```python
from build123d import *

# Parameters (mm, degrees)
SKETCH1_R           = 10
BOSS_EXTRUDE1_DEPTH = 10
SKETCH2_R           = 9.5
CUT_EXTRUDE1_DEPTH  = 6
SKETCH3_R           = 5
CUT_EXTRUDE2_DEPTH  = 11
CUT_EXTRUDE4_DEPTH  = 11
FILLET1_R           = 2
M4_TAPPED_HOLE1_D   = 3


with BuildPart() as part:
    # Sketch1 → Boss-Extrude1 (new body)
    with BuildSketch(Plane(origin=(0, 0, 0), x_dir=(1, 0, 0), z_dir=(0, 1, 0))):
        with BuildLine():
            Line((-14.758244484, -9.68540076), (-11.496273776, -137.792727273))
            ThreePointArc((-11.496273776, -137.792727273), (0, -149), (11.496273776, -137.792727273))
            Line((11.496273776, -137.792727273), (14.758244484, -9.68540076))
            ThreePointArc((14.758244484, -9.68540076), (15.434637081, -8.136753315), (17, -7.5))
            Line((17, -7.5), (17, 7.5))
            ThreePointArc((17, 7.5), (13.764151011, 8.182075624), (11.078928313, 10.112237509))
            ThreePointArc((11.078928313, 10.112237509), (0, 15), (-11.078928313, 10.112237509))
            ThreePointArc((-11.078928313, 10.112237509), (-13.764151011, 8.182075624), (-17, 7.5))
            Line((-17, 7.5), (-17, -7.5))
            ThreePointArc((-17, -7.5), (-15.434637081, -8.136753315), (-14.758244484, -9.68540076))
        make_face()
        Circle(SKETCH1_R, mode=Mode.SUBTRACT)
    extrude(amount=BOSS_EXTRUDE1_DEPTH)

    # Sketch2 → Cut-Extrude1 (cut)
    with BuildSketch(Plane(origin=(0, 0, 0), x_dir=(1, 0, 0), z_dir=(0, 1, 0))):
        with Locations((0, -137.5)):
            Circle(SKETCH2_R)
    extrude(amount=CUT_EXTRUDE1_DEPTH, mode=Mode.SUBTRACT)

    # Sketch3 → Cut-Extrude2 (cut, through all)
    with BuildSketch(Plane(origin=(0, 0, 0), x_dir=(-1, 0, 0), z_dir=(0, -1, 0))):
        with Locations((0, -137.5)):
            Circle(SKETCH3_R)
    extrude(amount=-CUT_EXTRUDE2_DEPTH, mode=Mode.SUBTRACT)

    # Sketch4 → Cut-Extrude4 (cut, through all)
    with BuildSketch(Plane(origin=(0, 0, 0), x_dir=(1, 0, 0), z_dir=(0, 1, 0))):
        with BuildLine():
            Line((-7.90050824, -82.580601653), (-6.96789079, -119.207272727))
            ThreePointArc((-6.96789079, -119.207272727), (0, -126), (6.96789079, -119.207272727))
            Line((6.96789079, -119.207272727), (7.90050824, -82.580601653))
            ThreePointArc((7.90050824, -82.580601653), (0, -74.476363636), (-7.90050824, -82.580601653))
        make_face()
        with BuildLine():
            Line((-9.376393506, -24.618181818), (-8.443776056, -61.244852893))
            ThreePointArc((-8.443776056, -61.244852893), (0, -69.476363636), (8.443776056, -61.244852893))
            Line((8.443776056, -61.244852893), (9.376393506, -24.618181818))
            ThreePointArc((9.376393506, -24.618181818), (0, -15), (-9.376393506, -24.618181818))
        make_face()
    extrude(amount=CUT_EXTRUDE4_DEPTH, mode=Mode.SUBTRACT)

    # Fillet1
    fillet1_edges = [part.edges().sort_by_distance(p)[0] for p in [
        (17, 5, -7.5),
        (17, 5, 7.5),
        (-17, 5, 7.5),
        (-17, 5, -7.5),
    ]]
    fillet(fillet1_edges, radius=FILLET1_R)

    # M4 Tapped Hole1 (through all)
    with Locations(Plane.ZY.offset(17)):
        with Locations((0, 5)):
            Hole(M4_TAPPED_HOLE1_D / 2)


solid = part.part
```
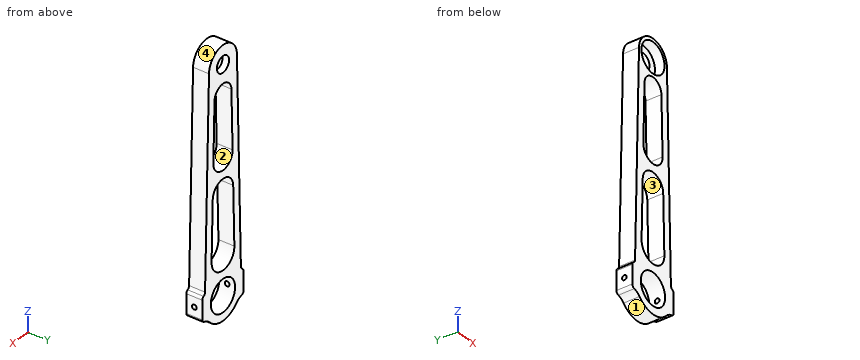
Geometry check sheet. Reference: the model listing, model coordinates, mm. Face numbers are marked on the shaded views. A direction names the side the tool comes from. Coordinates: 2 decimals unless noted, no trailing zeros. Order: outer loops, then holes, each group sorted by start corner. A loop starts at its lowest first (then second) coordinate and runs counter-clockwise, first axis right, second up.
Item 1: Scan lines: line 1 along Y through (x, z) = (-12, 0); line 2 along Z through (x, y) = (4, 9.5); line 3 along Z through (x, y) = (4.5, 6.5). Record each from-to range of solid material in increasing order.
Item 2: Tool access check on the marked faces 1 and 2. Record the directions out of +Z, -Z, +X, -X, +Y, -Y that give a thin tool (end or side, any length) a straight path to the whole face; none if there is none.
Item 3: Section check A-A (x = 0). Enter the section's corners in (y, z).
Item 4: Section check B-B (z = 0). Enter the section's corners in (x, y), plus the area to 3 significant figures.
Item 5: Section check D-D (x = 13). Enter the section's corners in (y, z).
Item 6: Mould release check, pull along X, two halves, no side actions. Record for the marked faces 3 and 4: released by +X, released by -X, zero draft, split by the parting line, or undercut.
Item 7: Depth check by flat-ended pin: pin 1 (1.5 mm diameter, centred on x = 12, y = 7, fed in from -Z); pin 2 (5.5 mm diameter, centred on x = -3.5, z = 133.5, fed in from -Y); pin 3 (1 mm diameter, centred on x = 13, y = 5.5, fed in from -Z). Enter the tip coordinate at first touch or a pass-through.
Item 8: Section check C-C (z = 100.5). Enter the section's corners in (x, y).
Check sheet entries:
1. line 1: y = 0 to 3.5, 6.5 to 10
1. line 2: z = -14.46 to -9.17, 9.17 to 15.9, 68.47 to 75.56, 124.74 to 134.5, 140.5 to 148.28
1. line 3: z = -14.31 to -8.93, 8.93 to 16.15, 68.18 to 75.88, 124.35 to 135.32, 139.68 to 148.08
2. face 1: -Z, +Y, -Y
2. face 2: +Y, -Y
3. outline: (0, -15) - (10, -15) - (10, -10) - (0, -10) - close; (0, 10) - (10, 10) - (10, 15) - (0, 15) - close; (0, 69.48) - (10, 69.48) - (10, 74.48) - (0, 74.48) - close; (0, 126) - (10, 126) - (10, 132.5) - (6, 132.5) - (6, 128) - (0, 128) - close; (0, 147) - (6, 147) - (6, 142.5) - (10, 142.5) - (10, 149) - (0, 149) - close
4. outline: (-17, 0) - (-10, 0) - (-10, 3.5) - (-17, 3.5) - close; (-17, 6.5) - (-10, 6.5) - (-10, 10) - (-17, 10) - close; (10, 0) - (17, 0) - (17, 3.5) - (10, 3.5) - close; (10, 6.5) - (17, 6.5) - (17, 10) - (10, 10) - close
4. area: 98.0 mm2
5. outline: (0, -8.57) - (10, -8.57) - (10, 78.74) - (0, 78.74) - close; hole circle Ø3 at (5, 0)
6. face 3: undercut
6. face 4: split by the parting line
7. pin 1: stops at z = -9.93
7. pin 2: stops at y = 6
7. pin 3: stops at z = -8.88
8. outline: (-12.45, 0) - (-7.44, 0) - (-7.44, 10) - (-12.45, 10) - close; (7.44, 0) - (12.45, 0) - (12.45, 10) - (7.44, 10) - close
